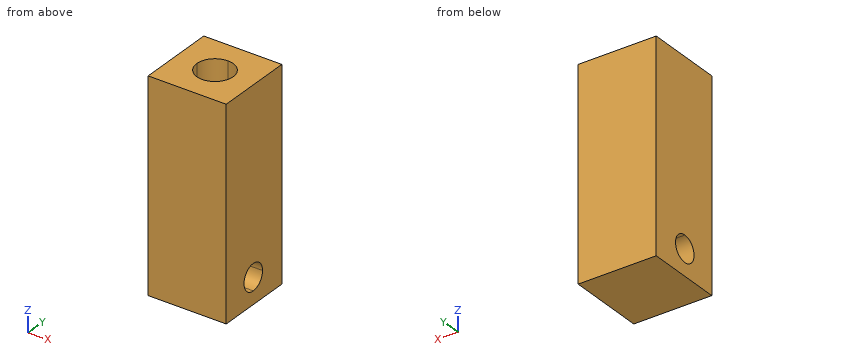
```python
from build123d import *

# Parameters (mm, degrees)
F1_DEPTH = 10
F2_DEPTH = 40
F4_DEPTH = 15


with BuildPart() as f1:
    # F0 (on Top) → F1 (new body)
    with BuildSketch(Plane.XY):
        with BuildLine():
            Line((7.5, 7.7042555064), (0, 7.7042555064))
            Line((0, 7.7042555064), (0, 3.7042555064))
            ThreePointArc((0, 3.7042555064), (2.4748737342, 2.6791292405), (3.5, 0.2042555064))
            Line((3.5, 0.2042555064), (7.5, 0.2042555064))
            Line((7.5, 0.2042555064), (7.5, 7.7042555064))
        make_face()
        with BuildLine():
            Line((0, 7.7042555064), (-7.5, 7.7042555064))
            Line((-7.5, 7.7042555064), (-7.5, 0.2042555064))
            Line((-7.5, 0.2042555064), (-3.5, 0.2042555064))
            ThreePointArc((-3.5, 0.2042555064), (-2.4748737342, 2.6791292405), (0, 3.7042555064))
            Line((0, 3.7042555064), (0, 7.7042555064))
        make_face()
        with BuildLine():
            Line((-3.5, 0.2042555064), (-7.5, 0.2042555064))
            Line((-7.5, 0.2042555064), (-7.5, -7.2957444936))
            Line((-7.5, -7.2957444936), (0, -7.2957444936))
            Line((0, -7.2957444936), (0, -3.2957444936))
            ThreePointArc((0, -3.2957444936), (-2.4748737342, -2.2706182278), (-3.5, 0.2042555064))
        make_face()
        with BuildLine():
            Line((7.5, -7.2957444936), (7.5, 0.2042555064))
            Line((7.5, 0.2042555064), (3.5, 0.2042555064))
            ThreePointArc((3.5, 0.2042555064), (2.4748737342, -2.2706182278), (0, -3.2957444936))
            Line((0, -3.2957444936), (0, -7.2957444936))
            Line((0, -7.2957444936), (7.5, -7.2957444936))
        make_face()
        with BuildLine():
            Line((0, 0.2042555064), (0, 3.7042555064))
            ThreePointArc((0, 3.7042555064), (-2.4748737342, 2.6791292405), (-3.5, 0.2042555064))
            Line((-3.5, 0.2042555064), (0, 0.2042555064))
        make_face()
        with BuildLine():
            ThreePointArc((3.5, 0.2042555064), (2.4748737342, 2.6791292405), (0, 3.7042555064))
            Line((0, 3.7042555064), (0, 0.2042555064))
            Line((0, 0.2042555064), (3.5, 0.2042555064))
        make_face()
        with BuildLine():
            Line((3.5, 0.2042555064), (0, 0.2042555064))
            Line((0, 0.2042555064), (0, -3.2957444936))
            ThreePointArc((0, -3.2957444936), (2.4748737342, -2.2706182278), (3.5, 0.2042555064))
        make_face()
        with BuildLine():
            Line((0, 0.2042555064), (-3.5, 0.2042555064))
            ThreePointArc((-3.5, 0.2042555064), (-2.4748737342, -2.2706182278), (0, -3.2957444936))
            Line((0, -3.2957444936), (0, 0.2042555064))
        make_face()
    extrude(amount=F1_DEPTH)

    # F0 (on Top) → F2 (join)
    with BuildSketch(Plane.XY):
        with BuildLine():
            Line((0, 7.7042555064), (-7.5, 7.7042555064))
            Line((-7.5, 7.7042555064), (-7.5, 0.2042555064))
            Line((-7.5, 0.2042555064), (-3.5, 0.2042555064))
            ThreePointArc((-3.5, 0.2042555064), (-2.4748737342, 2.6791292405), (0, 3.7042555064))
            Line((0, 3.7042555064), (0, 7.7042555064))
        make_face()
        with BuildLine():
            Line((7.5, 7.7042555064), (0, 7.7042555064))
            Line((0, 7.7042555064), (0, 3.7042555064))
            ThreePointArc((0, 3.7042555064), (2.4748737342, 2.6791292405), (3.5, 0.2042555064))
            Line((3.5, 0.2042555064), (7.5, 0.2042555064))
            Line((7.5, 0.2042555064), (7.5, 7.7042555064))
        make_face()
        with BuildLine():
            Line((-3.5, 0.2042555064), (-7.5, 0.2042555064))
            Line((-7.5, 0.2042555064), (-7.5, -7.2957444936))
            Line((-7.5, -7.2957444936), (0, -7.2957444936))
            Line((0, -7.2957444936), (0, -3.2957444936))
            ThreePointArc((0, -3.2957444936), (-2.4748737342, -2.2706182278), (-3.5, 0.2042555064))
        make_face()
        with BuildLine():
            Line((7.5, -7.2957444936), (7.5, 0.2042555064))
            Line((7.5, 0.2042555064), (3.5, 0.2042555064))
            ThreePointArc((3.5, 0.2042555064), (2.4748737342, -2.2706182278), (0, -3.2957444936))
            Line((0, -3.2957444936), (0, -7.2957444936))
            Line((0, -7.2957444936), (7.5, -7.2957444936))
        make_face()
    extrude(amount=F2_DEPTH)

    # F3 (on face) → F4 (cut)
    with BuildSketch(Plane.YZ.offset(7.5)):
        with BuildLine():
            ThreePointArc((0, 7.5), (-2.5, 5), (0, 2.5))
            Line((0, 2.5), (0, 5))
            Line((0, 5), (0, 7.5))
        make_face()
        with BuildLine():
            Line((0, 5), (0, 2.5))
            ThreePointArc((0, 2.5), (1.767766953, 3.232233047), (2.5, 5))
            ThreePointArc((2.5, 5), (1.767766953, 6.767766953), (0, 7.5))
            Line((0, 7.5), (0, 5))
        make_face()
    extrude(amount=-F4_DEPTH, mode=Mode.SUBTRACT)


solid = f1.part
```
Read the model definition and answer for the solid it produces. Units are mm, in the model's axes. Give positions to 0.01 mm unless a question says otherwise; leave off trailing zeros. Write each loop counter-clockwise with the first axis right and the second up, starting at its lowest first coordinate (ties: lowest second). Pieces come first, ordered by that corner, then holes. Notation, with made-up numbers: (43, -34.5) - (78, -34.5) arc R16 cw to (78, -20.5) - close; hole circle Ø5 at (39.25, 78.25). An arc over 180 degrees is marked (long way). Write item = value, one per line. Start each with the question number.
Item 1: Find section B-B (z = 36). Give the vertices of the cut face in (x, y), then the cut area to 3 significant figures.
Item 2: This flat-tipped pin is pushed along its axis until it touches: P1, Ø5.5, axis at x = 0.5, y = 0.5, coming from the +Z side. Where does it stop, or does it pass through?
Item 3: Find section A-A (x = -6.25). Give the vertices of the cut face in (y, z), then the cut area to 3 significant figures.
Item 4: Find section C-C (x = -1). Give the vertices of the cut face in (y, z).
Item 5: Find the intervals of material crossed by probe 1 along Z at (x, y) = (4, 2.25); probe 2 along Y at (x, z) = (0, 7); probe 3 along Z at (x, y) = (-3, 1.75), in increasing order. Write a range as [from, to].
Response:
q1.outline = (-7.5, -7.3) - (7.5, -7.3) - (7.5, 7.7) - (-7.5, 7.7) - close; hole circle Ø7 at (0, 0.2)
q1.area = 187 mm²
q2.P1 = 10
q3.outline = (-7.3, 0) - (7.7, 0) - (7.7, 40) - (-7.3, 40) - close; hole circle Ø5 at (0, 5)
q3.area = 580 mm²
q4.outline = (-7.3, 0) - (7.7, 0) - (7.7, 40) - (3.56, 40) - (3.56, 10) - (-3.15, 10) - (-3.15, 40) - (-7.3, 40) - close; hole circle Ø5 at (0, 5)
q5.probe_1 = [0, 3.91], [6.09, 40]
q5.probe_2 = [-7.3, -1.5], [1.5, 7.7]
q5.probe_3 = [0, 3.21], [6.79, 10]
